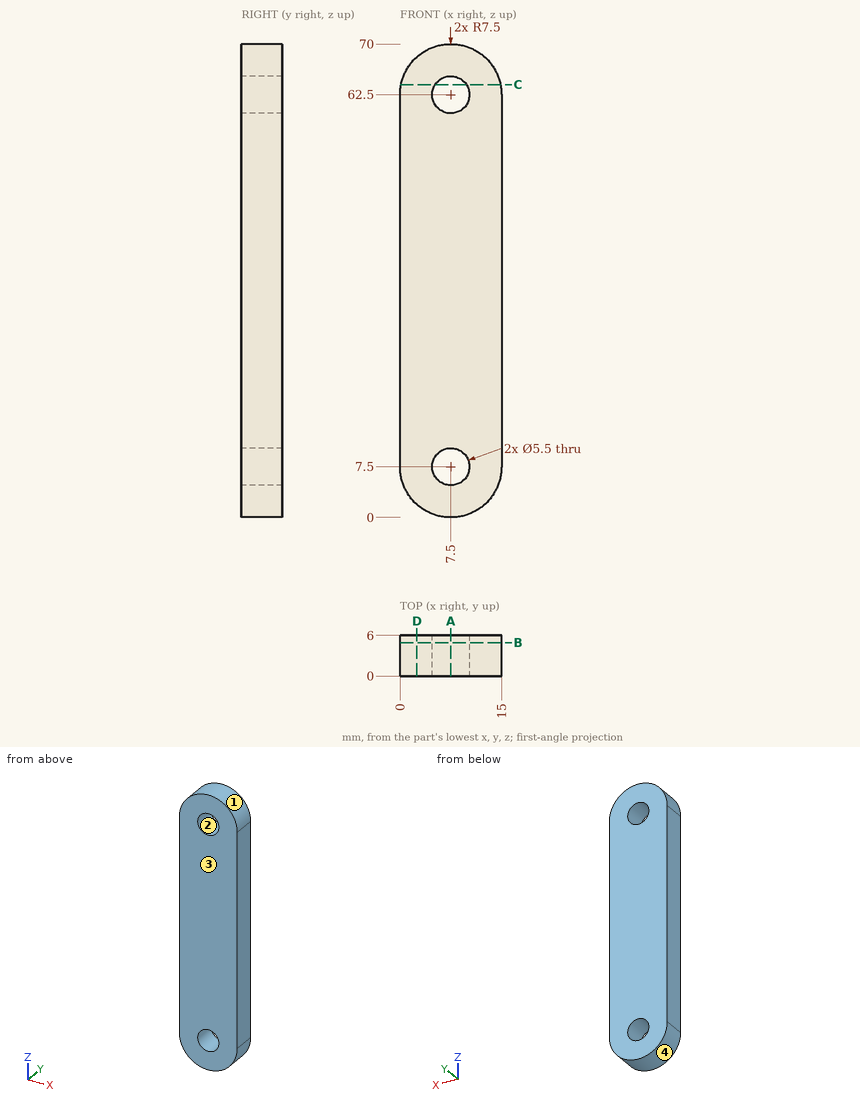
Geometry: see drawing. Coordinates: mm, zero at the bounding-box minimum. Give positions to 0.01 mm unless a question says otherwise; leave off trailing zeros. Loops run counter-clockwise (first coordinate to the right, second up) from the corner with the lowest first, then second, coordinate; pieces in that order, holes last. Notation, with made-up numbers: M 64.25,73 L 103.25,73 A21 ccw 103.25,89 Z; hole C 30.25,-17 d6. An arc over 180 degrees is marked long. Use one line per item in the form item = value.
1. Section query B-B, the plane y = 4.95. Return the cut outline in (x, z).
Numbers:
outline = M 0,7.5 A7.5 ccw 15,7.5 L 15,62.5 A7.5 ccw 0,62.5 Z; hole C 7.5,7.5 d5.5; hole C 7.5,62.5 d5.5
2. Pull-direction query (Z, two-part tool) for the marked faces 1, 2, 3 and 4; classes: released by +Z, released by -Z, zero draft, split by the parting line, or undercut.
Numbers:
face_1 = released by +Z
face_2 = undercut
face_3 = zero draft
face_4 = released by -Z
3. Section query D-D, the plane x = 2.5. Return the cut outline in (y, z), and give its area (3 significant figures).
Numbers:
outline = M 0,1.91 L 6,1.91 L 6,68.09 L 0,68.09 Z
area = 397 mm²
4. Section query A-A, the plane x = 7.5. Return the cut outline in (y, z).
Numbers:
outline = M 0,0 L 6,0 L 6,4.75 L 0,4.75 Z; M 0,10.25 L 6,10.25 L 6,59.75 L 0,59.75 Z; M 0,65.25 L 6,65.25 L 6,70 L 0,70 Z
5. Section query C-C, the plane z = 64. Return the cut outline in (x, y), and give its area (3 significant figures).
Numbers:
outline = M 0.15,0 L 5.2,0 L 5.2,6 L 0.15,6 Z; M 9.8,0 L 14.85,0 L 14.85,6 L 9.8,6 Z
area = 60.5 mm²
6. First-contact query: pin 1 (3.5 mm diameter, centred on x = 7.5, z = 7.5, fed in from +Y). Flat tip, straight axial feed; report the tip coordinate or a pass-through.
Numbers:
pin_1 = through
7. Line query: L1, parallel to Z at x = 7.5, y = 3.8; L2, parallel to Z at x = 9.5, y = 3.6; L3, parallel to Z at x = 4, y = 2.4. Output: solid intervals per line, ascending.
Numbers:
L1 = 0 to 4.75, 10.25 to 59.75, 65.25 to 70
L2 = 0.27 to 5.61, 9.39 to 60.61, 64.39 to 69.73
L3 = 0.87 to 69.13
